Input: part model. Units: mm. Frame: model coordinates. A direction names the side the tool comes from. Give positions to 0.01 mm unless a question says otherwise; leave off trailing zeros. Order: outer loops, then holes, each group sorted by start corner. A loop starts at its lowest first (then second) coordinate and runs counter-clockwise, first axis right, second up. Notation, with made-up numbers: (63.5, -20) - (121.5, -20) arc R20 cw to (121.5, 16) - close; hole circle Ø11 at (43, 29.5). An arc over 180 degrees is marked (long way). Use a Markdown table: item, result.
from build123d import *

# Parameters (mm, degrees)
SKETCH1_R               = 3.048
BOSS_EXTRUDE1_DEPTH     = 33.02
CUT_EXTRUDE1_DEPTH      = 5.953
CUT_EXTRUDE1_DEPTH_BACK = 5.953


with BuildPart() as part:
    # Sketch1 → Boss-Extrude1 (new body)
    with BuildSketch(Plane(origin=(0, 0, 0), x_dir=(1, 0, 0), z_dir=(0, 1, 0))):
        Circle(SKETCH1_R)
    extrude(amount=BOSS_EXTRUDE1_DEPTH)

    # Sketch2 → Revolve3 (revolve)
    with BuildSketch(Plane.XY):
        with BuildLine():
            Line((0, 37.973), (0, 35.941))
            ThreePointArc((0, 35.941), (-2.921, 33.02), (0, 30.099))
            Line((0, 30.099), (0, 28.067))
            ThreePointArc((0, 28.067), (-4.953, 33.02), (0, 37.973))
        make_face()
    revolve(axis=Axis((0, 37.973, 0), (0, -1, 0)))

    # Sketch3 → Cut-Extrude1 (cut, two sides)
    with BuildSketch(Plane(origin=(0, 0, 0), x_dir=(0, 0, -1), z_dir=(1, 0, 0))) as cut_extrude1_sk:
        with BuildLine():
            Line((-2.032, 37.973), (-2.032, 29.845))
            ThreePointArc((-2.032, 29.845), (-2.478369265, 28.767369265), (-3.556, 28.321))
            Line((-3.556, 28.321), (-6.35, 28.321))
            Line((-6.35, 28.321), (-6.35, 37.973))
            Line((-6.35, 37.973), (-2.032, 37.973))
        make_face()
        with BuildLine():
            Line((6.35, 37.973), (2.032, 37.973))
            Line((2.032, 37.973), (2.032, 29.845))
            ThreePointArc((2.032, 29.845), (2.478369265, 28.767369265), (3.556, 28.321))
            Line((3.556, 28.321), (6.35, 28.321))
            Line((6.35, 28.321), (6.35, 37.973))
        make_face()
    extrude(amount=CUT_EXTRUDE1_DEPTH, mode=Mode.SUBTRACT)
    extrude(cut_extrude1_sk.sketch, amount=-CUT_EXTRUDE1_DEPTH_BACK, mode=Mode.SUBTRACT)

    # Sketch4 → Cut-Revolve1 (revolve, cut)
    with BuildSketch(Plane.XY):
        with BuildLine():
            Line((0, 35.941), (0, 30.099))
            ThreePointArc((0, 30.099), (-2.921, 33.02), (0, 35.941))
        make_face()
    revolve(axis=Axis((0, 35.941, 0), (0, -1, 0)), mode=Mode.SUBTRACT)

    # Mirror1: part across plane


with BuildPart() as part_1:
    add(part.part)
    add(part.part.mirror(Plane.ZX))


solid = part_1.part
1. Section query B-B (y = 2). Return loops of the section in (x, z), then the cut area to 3 significant figures.
Response:
| item | result |
|---|---|
| outline | circle Ø6.1 at (0, 0) |
| area | 29.2 mm^2 |
2. Set-up query: faces 1 (the face through (0.1, 35.5, 2.032)), 2 (the face through (0.1, -35.5, 2.032)), 3 (the face through (-0.1, -35.5, -2.032)), 4 (the face through (-0.1, 35.5, -2.032)). Return all of +Z, -Z, +X, -X, +Y, -Y with unobstructed straight access to the full face (end or side cutting, diameter ignored); none if empty.
Response:
| item | result |
|---|---|
| face 1 | +Z, +X, -X, +Y |
| face 2 | +Z, +X, -X, -Y |
| face 3 | -Z, +X, -X, -Y |
| face 4 | -Z, +X, -X, +Y |
3. Pin query (flat end, axial travel): pin 1 (4 mm diameter, centred on x = 2, y = -34, fed in from +Z); pin 2 (1.5 mm diameter, centred on x = -3.5, y = -21.5, fed in from -Z); pin 3 (1 mm diameter, centred on x = -0.5, z = -1, fed in from +Y). Return the tip coordinate at first contact, or that it passes through.
Response:
| item | result |
|---|---|
| pin 1 | stops at z = 2.03 |
| pin 2 | stops at z = -1.31 |
| pin 3 | stops at y = 37.93 |
4. Material intervals for line 1 along Y through (x, z) = (2.25, 1); line 2 along Y through (x, z) = (-1.25, 1.75); line 3 along Y through (x, z) = (3.75, 1), sorted ascending.
Response:
| item | result |
|---|---|
| line 1 | y = -37.32 to -34.59, -31.45 to 31.45, 34.59 to 37.32 |
| line 2 | y = -37.48 to -35, -31.04 to 31.04, 35 to 37.48 |
| line 3 | y = -36.1 to -29.94, 29.94 to 36.1 |
5. Section query A-A (z = 0). Return loops of the section in (x, y), then the cut area to 3 significant figures.
Response:
| item | result |
|---|---|
| outline | (-3.05, -29.12) arc R4.95 ccw (long way) to (3.05, -29.12) - (3.05, 29.12) arc R4.95 ccw (long way) to (-3.05, 29.12) - close; hole circle Ø5.84 at (0, -33.02); hole circle Ø5.84 at (0, 33.02) |
| area | 447 mm^2 |
